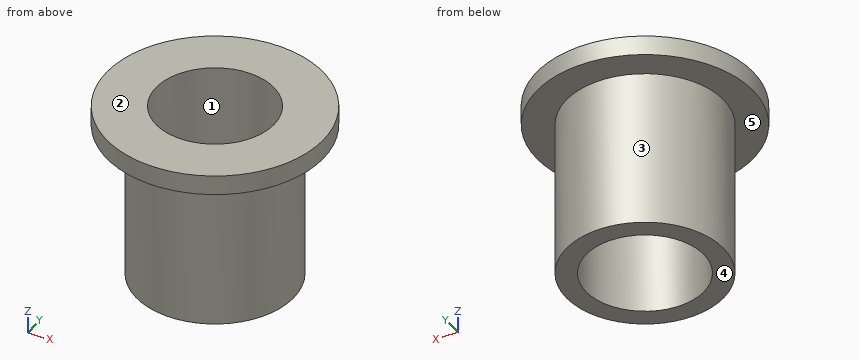
from build123d import *

# Parameters (mm, degrees)
SKETCH1_R           = 8.73125
BOSS_EXTRUDE1_DEPTH = 1.5875
SKETCH2_R           = 6.35
BOSS_EXTRUDE2_DEPTH = 12.7
SKETCH3_R           = 4.7625
CUT_EXTRUDE1_DEPTH  = 15.2875


with BuildPart() as part:
    # Sketch1 → Boss-Extrude1 (new body)
    with BuildSketch(Plane.XY):
        Circle(SKETCH1_R)
    extrude(amount=BOSS_EXTRUDE1_DEPTH)

    # Sketch2 → Boss-Extrude2 (add)
    with BuildSketch(Plane(origin=(0, 0, 0), x_dir=(-1, 0, 0), z_dir=(0, 0, -1))):
        Circle(SKETCH2_R)
    extrude(amount=BOSS_EXTRUDE2_DEPTH)

    # Sketch3 → Cut-Extrude1 (cut, through all)
    with BuildSketch(Plane.XY.offset(1.5875)):
        Circle(SKETCH3_R)
    extrude(amount=-CUT_EXTRUDE1_DEPTH, mode=Mode.SUBTRACT)


solid = part.part
The listing builds one solid part. Answer for the finished solid, in the listing's coordinates (mm). Face numbers are marked on the shaded views. A direction names the side the tool comes from. Give positions to 0.01 mm unless a question says otherwise; leave off trailing zeros. Write each loop counter-clockwise with the first axis right and the second up, starting at its lowest first coordinate (ties: lowest second). Pieces come first, ordered by that corner, then holes. Notation, with made-up numbers: (89.5, 7) - (98.5, 7) arc R19 cw to (98.5, 22) - close; hole circle Ø2 at (-9, 57). An arc over 180 degrees is marked (long way). One line per question, with ' | ' between items. Start each with the question number.
1. Given P1, Ø2, axis at y = 4.5, z = -5, coming from the -X side; P2, Ø5, axis at x = -5.5, z = -3, coming from the +Y side; P3, Ø8, axis at x = 5, z = -6, coming from the +Y side, each flat-ended and moving along its own axis, determine where each tip first touches the part or whether it passes through.
2. Determine the mould class of the marked faces 1, 2 and 3 for opening direction Y: +Y half, -Y half, draft (parallel to the pull), parting line (faces both ways), or undercut.
3. For the marked faces 4 and 5, determine the directions among +Z, -Z, +X, -X, +Y, -Y from which every point of the face is accessible in a straight line to the end or side of a thin tool.
4. Section A-A, the plane y = 0 is taken. Determine the outline of the cut face in (x, z).
5. Section D-D, the plane x = 5.25 is taken. Determine the outline of the cut face in (y, z).
6. Straight lines are drawn through the part: line 1 (Y direction, x = 0, z = -6.5); line 2 (Z direction, x = -5.75, y = 6.5); line 3 (Y direction, x = 2.75, z = -0.25). For each, find the intervals that lie inside material, in ascending order.
Result:
1) P1: stops at x = -5.3 | P2: stops at y = 5.6 | P3: stops at y = 6.27
2) face 1: undercut | face 2: draft | face 3: parting line
3) face 4: -Z, +X, -X, +Y, -Y | face 5: -Z
4) outline: (-8.73, 0) - (-6.35, 0) - (-6.35, -12.7) - (-4.76, -12.7) - (-4.76, 1.59) - (-8.73, 1.59) - close; (4.76, -12.7) - (6.35, -12.7) - (6.35, 0) - (8.73, 0) - (8.73, 1.59) - (4.76, 1.59) - close
5) outline: (-6.98, 0) - (-3.57, 0) - (-3.57, -12.7) - (3.57, -12.7) - (3.57, 0) - (6.98, 0) - (6.98, 1.59) - (-6.98, 1.59) - close
6) line 1: y = -6.35 to -4.76, 4.76 to 6.35 | line 2: z = 0 to 1.59 | line 3: y = -5.72 to -3.89, 3.89 to 5.72
